Geometry: final body of the model. Coordinates: model frame, mm. A direction names the side the tool comes from. Round coordinates to 2 decimals unless told otherwise and drop trailing zeros. Loops run counter-clockwise (first coordinate to the right, second up) from the corner with the lowest first, then second, coordinate; pieces in that order, holes last. Notation, with made-up numbers: (-11, 84.5) -> (13, 84.5) arc R30 cw to (13, 108.5) -> close; hole circle Ø10 at (50, 30.5). An arc over 180 degrees is marked (long way). Answer in a Markdown table with one row per item.
Autodesk Inventor part; units mm, degrees
ref_plane "YZ Plane" through (0, 0, 0) normal (1, 0, 0) x (0, 1, 0)
ref_plane "XZ Plane" through (0, 0, 0) normal (0, 1, 0) x (-1, 0, 0)
ref_plane "XY Plane" through (0, 0, 0) normal (0, 0, 1) x (1, 0, 0)
sketch "Sketch1" plane through (0, 0, 0) normal (0, 1, 0) x (-1, 0, 0)
  circle A0 centre (0, 0) radius 2.7
  dimension "headDiameter" = 5.4
extrude "Extrusion1" add sketch "Sketch1" along normal blind 2
sketch "Sketch2" plane through (0, 2, 0) normal (0, 1, 0) x (1, 0, 0)
  line L0 (0.5, -2.7) -> (-0.5, -2.7)
  line L1 (-0.5, -2.7) -> (-0.5, 2.7)
  line L2 (-0.5, 2.7) -> (0.5, 2.7)
  line L3 (0.5, 2.7) -> (0.5, -2.7)
  line L4 (0.5, -2.7) -> (-0.5, 2.7) construction
  line L5 (-0.5, -2.7) -> (0.5, 2.7) construction
  point P0 (0, 0)
  dimension "d3" = 1
  dimension "d4" = 5.4
extrude "Extrusion2" cut sketch "Sketch2" against normal blind 0.75
sketch "Sketch3" plane through (0, 0, 0) normal (0, -1, 0) x (1, 0, 0)
  circle A0 centre (0, 0) radius 1.5
  dimension "d7" = 3
extrude "Extrusion3" add sketch "Sketch3" along normal blind 15
chamfer "Chamfer1" distance 0.5 angle 45 1 edges at (-1.5, -15, 0)
fillet "Fillet1" radius 0.5 3 edges at (-2.0785, 2, 1.7234) (-2.0785, 2, -1.7234) (2.7, 2, 0)
equation "\"d4\" = headDiameter"
properties part number "machineScrew3x15" material "Stainless Steel"
Item 1: Section query A-A, the plane z = 0. Output: boundary loops of the cut face in (x, y).
Ans:
| item | result |
|---|---|
| outline | (-2.7, 0) -> (-1.5, 0) -> (-1.5, -14.5) -> (-1, -15) -> (1, -15) -> (1.5, -14.5) -> (1.5, 0) -> (2.7, 0) -> (2.7, 1.5) arc R0.5 ccw to (2.2, 2) -> (0.5, 2) -> (0.5, 1.25) -> (-0.5, 1.25) -> (-0.5, 2) -> (-2.2, 2) arc R0.5 ccw to (-2.7, 1.5) -> close |
Item 2: Mould query, pull axis X, two halves, no side actions, for faces 3 (the cylindrical face through (-1.5, -7.15, -0.07)), 4 (the flat face through (0, 1.25, 0)), 5 (the flat face through (-1, 2, 0)). Classes: released by +X, released by -X, zero draft, split by the parting line, or undercut.
Ans:
| item | result |
|---|---|
| face 3 | split by the parting line |
| face 4 | undercut |
| face 5 | zero draft |
Item 3: Set-up query: faces 1 (the flat face through (-1.2, 0, -1.2)), 2 (the flat face through (1, 2, 0)). Return all of +Z, -Z, +X, -X, +Y, -Y with unobstructed straight access to the full face (end or side cutting, diameter ignored); none if empty.
Ans:
| item | result |
|---|---|
| face 1 | -Y |
| face 2 | +Z, -Z, +X, -X, +Y |
Item 4: First-contact query: P1, Ø1.1, axis at x = 0, z = -1, coming from the +Y side; P2, Ø1.5, axis at x = 1, y = -11.5, coming from the +Z side; P3, Ø0.6, axis at y = 2, z = -0.5, coming from the +X side; P4, Ø0.8, axis at y = 1.5, z = -0.5, coming from the -X side. Flat tips, straight axial feed; report the tip coordinate or a pass-through.
Ans:
| item | result |
|---|---|
| P1 | y = 2 |
| P2 | z = 1.48 |
| P3 | x = 2.62 |
| P4 | x = -2.7 |
Item 5: Ray query, L1, parallel to Y at x = 2.15, z = 0.4; L2, parallel to Y at x = -0.35, z = -0.25; L3, parallel to Z at x = 0.65, y = -3.25. Return the intervals inside material, ascending.
Ans:
| item | result |
|---|---|
| L1 | 0 to 2 |
| L2 | -15 to 1.25 |
| L3 | -1.35 to 1.35 |
Item 6: Section query B-B, the plane x = 0. Output: boundary loops of the cut face in (y, z).
Ans:
| item | result |
|---|---|
| outline | (-15, -1) -> (-14.5, -1.5) -> (0, -1.5) -> (0, -2.7) -> (1.25, -2.7) -> (1.25, 2.7) -> (0, 2.7) -> (0, 1.5) -> (-14.5, 1.5) -> (-15, 1) -> close |
Item 7: Section query C-C, the plane y = 0.25. Output: boundary loops of the cut face in (x, z), and give its area (3 significant figures).
Ans:
| item | result |
|---|---|
| outline | circle Ø5.4 at (0, 0) |
| area | 22.9 mm2 |
